from build123d import *

# Parameters (mm, degrees)
SKETCH_R  = 2.05
PAD_DEPTH = 4
FILLET_R  = 1


with BuildPart() as part:
    # Sketch → Pad (new body)
    with BuildSketch(Plane.XY):
        with BuildLine():
            Line((0, 5), (-7, 5))
            Line((-7, 5), (-7, -5))
            Line((0, -5), (-7, -5))
            ThreePointArc((0, -5), (5, 0), (0, 5))
        make_face()
        Circle(SKETCH_R, mode=Mode.SUBTRACT)
    extrude(amount=PAD_DEPTH)

    # AdditivePipe: sweep along a path in Sketch001
    with BuildLine(Plane.XZ) as additivepipe_path:
        ThreePointArc((-7, 0), (-12.8578643763, 14.1421356237), (-27, 20))
        Line((-27, 20), (-110, 20))
    # Sketch002 → AdditivePipe (sweep)
    with BuildSketch(Plane.XY):
        Polygon((-8.443375673, -2.5), (-5.556624327, -2.5), (-4.1132486541, 0), (-5.556624327, 2.5), (-8.443375673, 2.5), (-9.8867513459, 0), align=None)
    sweep(path=additivepipe_path.line, is_frenet=True)

    # Sketch003 (on Face22 of AdditivePipe) → Revolution (revolve)
    with BuildSketch(Plane(origin=(-107.7, 0, 0), x_dir=(0, -1, 0), z_dir=(-1, 0, 0))):
        Polygon((0, 20), (-3.4202014333, 10.6030737921), (-1.5408161917, 9.9190335055), (2.1612930278, 19.2133536704), align=None)
    revolve(axis=Axis((-107.7, 6.4278760969, 2.3395555688), (0, 0.3420201433, -0.9396926208)))

    # Fillet
    fillet_edges = [part.edges().sort_by_distance(p)[0] for p in [
        (-6.466502, 2.5, 4),
        (-5.198955, 1.250176, 4),
        (-5.198955, -1.250176, 4),
        (-6.466502, -2.5, 4),
        (-7, -2.5, 2),
        (-7, -5, 2),
        (-7, 2.5, 2),
        (-7, 5, 2),
    ]]
    fillet(fillet_edges, radius=FILLET_R)


solid = part.part
Part model, mm, in its own coordinate system. A direction names the side the tool comes from. Round coordinates to 2 decimals unless told otherwise and drop trailing zeros. Loops run counter-clockwise (first coordinate to the right, second up) from the corner with the lowest first, then second, coordinate; pieces in that order, holes last. Notation, with made-up numbers: (77, -21.75) - (112, -21.75) arc R21 cw to (112, 2.25) - close; hole circle Ø10 at (79.25, 15.5). An arc over 180 degrees is marked (long way). Answer as a JSON object with one key per item and string values.
Item 1: Pull direction Y, two halves, no side cores. Call faces 1 (the face through (-14.6, 0.4, 12.13)), 2 (the face through (-0.267, 2.033, 1.972)), 3 (the face through (-3, 0, 0)), 4 (the face through (-69.081, -1.232, 17.825)): pulls with the +Y half, pulls with the -Y half, needs draft (parallel to the pull), parting line crosses it, or undercut.
Output:
{"face 1": "pulls with the +Y half", "face 2": "undercut", "face 3": "needs draft", "face 4": "pulls with the -Y half"}
Item 2: Pin check, flat tips, straight feed: pin 1 (1.5 mm diameter, centred on y = -3, z = 7.5, fed in from +X); pin 2 (5 mm diameter, centred on y = -1, z = 19.5, fed in from +X); pin 3 (2 mm diameter, centred on y = 0, z = 18.5, fed in from +X). Stop position of each tip, or through.
Output:
{"pin 1": "x = -6.68", "pin 2": "x = -11.91", "pin 3": "x = -12.25"}
Item 3: Tool access for faces 5 (the face through (-14.59, -0.43, 12.14)), 6 (the face through (-2.4, 0.1, 4)), 7 (the face through (5, 0, 2)): list every direction of +Z, -Z, +X, -X, +Y, -Y with a clear straight run to the whole face (end or side of a thin tool).
Output:
{"face 5": "-Z, -Y", "face 6": "+Z, +X", "face 7": "+Z, -Z, +X"}
Item 4: Band-saw the part on A-A on x = -44. List the corners of the cut face in (y, z), plus the area to 3 significant figures.
Output:
{"outline": "(-2.5, 18.56) - (0, 17.11) - (2.5, 18.56) - (2.5, 21.44) - (0, 22.89) - (-2.5, 21.44) - close", "area": "21.7 mm2"}
Item 5: Wall check: L1, parallel to Z at x = -66, y = 0.25; L2, parallel to Z at x = -105, y = -0.75; L3, parallel to Y at x = -94.5, z = 17.5. Give the ranges that are in metal, low to high.
Output:
{"L1": "17.26 to 22.74", "L2": "17.55 to 22.45", "L3": "-0.67 to 0.67"}
